Source: CAD feature listing. Evaluate the final solid. Frame: model axes, mm. A direction names the side the tool comes from. Give positions to 0.01 mm unless a question says otherwise; leave off trailing zeros. Order: outer loops, then holes, each group sorted by start corner. A loop starts at its lowest first (then second) coordinate and runs counter-clockwise, first axis right, second up. Notation, with made-up numbers: (8.5, 70) - (52.5, 70) arc R5 ccw to (52.5, 75) - close; hole circle Ø10 at (57.25, 70.25). An arc over 180 degrees is marked (long way). Answer as CSV lines item,"result".
```python
from build123d import *

# Parameters (mm, degrees)
F0_W     = 152.4
F0_H     = 127
F1_DEPTH = 152.4
F2_T     = -2.54
F3_W     = 144.78
F3_H     = 4.651744
F3_W_2   = 149.86
F3_H_2   = 4.752902
F4_DEPTH = 152.4
F5_W     = 152.4
F5_H     = 4.3434
F6_DEPTH = 152.4
F8_DEPTH = 152.4


with BuildPart() as f1:
    # F0 (on Front) → F1 (new body)
    with BuildSketch(Plane.XZ):
        with Locations((-40.71237, -4.145074)):
            Rectangle(F0_W, F0_H)
    extrude(amount=F1_DEPTH)

    # F2
    f2_openings = [f1.faces().sort_by_distance(p)[0] for p in [
        (-40.71237, -152.4, -4.145074),
    ]]
    offset(amount=F2_T, openings=f2_openings)

    # F3 (on Front) → F4 (join)
    with BuildSketch(Plane.XZ):
        with Locations((-41.570326, 15.118169)):
            Rectangle(F3_W, F3_H)
        with Locations((-39.960672, -27.394711)):
            Rectangle(F3_W_2, F3_H_2)
    extrude(amount=F4_DEPTH)

    # F5 (on Front) → F6 (join)
    with BuildSketch(Plane.XZ):
        with Locations((-41.850881, 14.875366)):
            Rectangle(F5_W, F5_H)
    extrude(amount=F6_DEPTH)

    # F7 (on Front) → F8 (join)
    with BuildSketch(Plane.XZ):
        Polygon((-38.857852, 59.844222), (-41.029552, 59.844222), (-43.201252, 59.844222), (-43.201252, -24.935095), (-38.857852, -24.935095), align=None)
    extrude(amount=F8_DEPTH)


solid = f1.part
```
(1) Access query for faces 1 (the flat face through (-59, -152.4, 15)), 2 (the flat face through (-81, -75, 59.355)), 3 (the flat face through (-118.051, -75, 15)), 4 (the flat face through (-2, -75, 59.355)), 5 (the flat face through (-42, -76, -65.105)). Directions: +Z, -Z, +X, -X, +Y, -Y. A direction counts if a zero-diameter tool reaches every point of the face in a straight line with its end or side. Return the directions, or none.
Completed:
face 1,"+Z, -Z, +X, -X, -Y"
face 2,"+Z, -X, +Y, -Y"
face 3,"+Z, -Z, -X, +Y, -Y"
face 4,"+Z, +X, +Y, -Y"
face 5,"-Y"
(2) Mould query, pull axis X, two halves, no side actions, for faces 6 (the flat face through (-116.912, -75, 38)), 7 (the flat face through (-41, -75, 59.844)), 8 (the flat face through (-114.372, -76, -48)). Classes: released by +X, released by -X, zero draft, split by the parting line, or undercut.
Completed:
face 6,"released by -X"
face 7,"zero draft"
face 8,"undercut"
(3) Cut plane A-A (x = -35). Return loops of the section in (y, z), then the cut area to 3 significant figures.
Completed:
outline,"(-152.4, -67.65) - (0, -67.65) - (0, 59.35) - (-152.4, 59.35) - (-152.4, 56.81) - (-2.54, 56.81) - (-2.54, 17.44) - (-152.4, 17.44) - (-152.4, 12.7) - (-2.54, 12.7) - (-2.54, -25.02) - (-152.4, -25.02) - (-152.4, -29.77) - (-2.54, -29.77) - (-2.54, -65.11) - (-152.4, -65.11) - close"
area,"2,510 mm²"
(4) Contact query for flat-ended pins moving along their axis: pin 1 (1 mm diameter, centred on x = -71.5, y = -90, fed in from +Z); pin 2 (3 mm diameter, centred on x = -4.5, z = 10.5, fed in from -Y); pin 3 (3 mm diameter, centred on x = -11, z = 33.5, fed in from +Y); pin 4 (6 mm diameter, centred on y = -42.5, z = 30.5, fed in from -X). Output: stop coordinate, or through.
Completed:
pin 1,"z = 59.35"
pin 2,"y = -2.54"
pin 3,"y = 0"
pin 4,"x = -116.91"
(5) Cut plane C-C (y = -95). Give the number of separate pieces and of enclosed holes in the cut face, then the cut area to 3 significant figures.
Completed:
separate pieces,"1"
enclosed holes,"4"
area,"3,130 mm²"
(6) Cut plane B-B (z = 39). Return loops of the section in (x, y), then the cut area to 3 significant figures.
Completed:
outline,"(-116.91, -152.4) - (-114.37, -152.4) - (-114.37, -2.54) - (-43.2, -2.54) - (-43.2, -152.4) - (-38.86, -152.4) - (-38.86, -2.54) - (32.95, -2.54) - (32.95, -152.4) - (35.49, -152.4) - (35.49, 0) - (-116.91, 0) - close"
area,"1,800 mm²"
(7) Ray query, line 1 (Z direction, x = 28, y = -21); line 2 (X direction, y = -85, z = 8); line 3 (X direction, y = -99, z = -57). Return the intervals inside material, ascending. Write a range as from..to.
Completed:
line 1,"-67.65..-65.11, -29.77..-25.02, 12.7..17.44, 56.81..59.35"
line 2,"-116.91..-114.37, -43.2..-38.86, 32.95..35.49"
line 3,"-116.91..-114.37, 32.95..35.49"
